```python
from build123d import *

# Parameters (mm, degrees)
BOSS_EXTRUDE1_DEPTH = 35
SKETCH5_R           = 1.5
BOSS_EXTRUDE2_DEPTH = 8.091605471
SKETCH6_R           = 1.5
CUT_EXTRUDE1_DEPTH  = 4


with BuildPart() as part:
    # Sketch3 → Boss-Extrude1 (new body)
    with BuildSketch(Plane(origin=(0, 0, 0), x_dir=(1, 0, 0), z_dir=(0, 1, 0))):
        Polygon((-3.464101615, 0), (-1.732050808, -3), (1.732050808, -3), (3.464101615, 0), (1.732050808, 3), (-1.732050808, 3), align=None)
    extrude(amount=BOSS_EXTRUDE1_DEPTH)

    # Sketch5 → Boss-Extrude2 (add)
    with BuildSketch(Plane(origin=(0, 35, 0), x_dir=(1, 0, 0), z_dir=(0, 1, 0))):
        with Locations(Location((0, 0, 0), (0, 0, 270))):
            Circle(SKETCH5_R)
    extrude(amount=BOSS_EXTRUDE2_DEPTH)

    # Sketch6 → Cut-Extrude1 (cut)
    with BuildSketch(Plane.XZ):
        with Locations(Location((0, 0, 0), (0, 0, 90))):
            Circle(SKETCH6_R)
    extrude(amount=-CUT_EXTRUDE1_DEPTH, mode=Mode.SUBTRACT)


solid = part.part
```
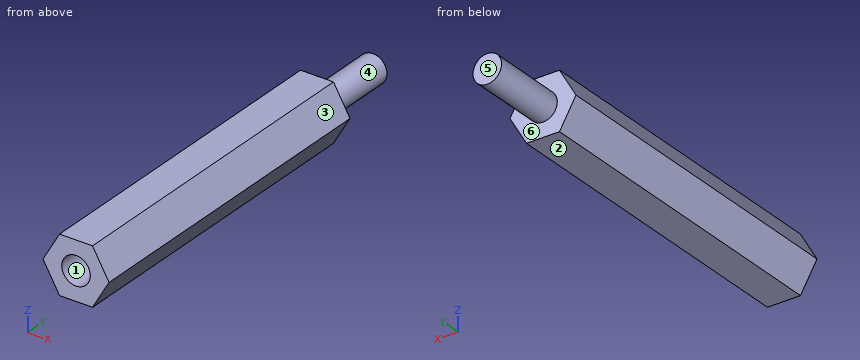
Can you work these out from the model? Positions are in its coordinate system, mm. Face numbers are marked on the shaded views. A direction names the side the tool comes from. Give positions to 0.01 mm unless a question says otherwise; leave off trailing zeros. Order: outer loops, then holes, each group sorted by start corner. A loop starts at its lowest first (then second) coordinate and runs counter-clockwise, first axis right, second up. Notation, with made-up numbers: M 56,-34.75 L 87,-34.75 A17 ccw 87,-1.75 Z; hole C -29.75,40 d4. An arc over 180 degrees is marked long. One line per item, written item: value.
1) I want a section at A-A, the plane x = 0. List the corners of the cut face in (y, z) for me.
Answer sheet:
outline: M 0,-3 L 35,-3 L 35,-1.5 L 43.09,-1.5 L 43.09,1.5 L 35,1.5 L 35,3 L 0,3 L 0,1.5 L 4,1.5 L 4,-1.5 L 0,-1.5 Z
2) I want a section at C-C, the plane z = 2. List the corners of the cut face in (x, y) for me, plus the area to 3 significant figures.
Answer sheet:
outline: M -2.31,0 L 2.31,0 L 2.31,35 L -2.31,35 Z
area: 162 mm^2
3) Please list where these lines run through material, in increasing order: line 1 along X through (y, z) = (1.45, 0); line 2 along Y through (x, z) = (2.75, 1); line 3 along Y through (x, z) = (-0.25, 0.75).
Answer sheet:
line 1: x = -3.46 to -1.5, 1.5 to 3.46
line 2: y = 0 to 35
line 3: y = 4 to 43.09
4) On a 3-axis mill with a long thin cutter (end or side, diameter ignored), from which of +Z, -Z, +X, -X, +Y, -Y can I reach the whole of each face in a straight line? I mean the marked faces 5 and 6. Say none if no direction works.
Answer sheet:
face 5: +Z, -Z, +X, -X, +Y
face 6: +Y
5) I want a section at D-D, the plane x = -3. List the corners of the cut face in (y, z) for me, plus the area to 3 significant figures.
Answer sheet:
outline: M 0,-0.8 L 35,-0.8 L 35,0.8 L 0,0.8 Z
area: 56.3 mm^2
6) For P1, Ø2, axis at x = -2.5, z = 1, coming from the +Y side, with a flat end and sliding along its axis, tell me the tip position at first contact or that it passes through.
Answer sheet:
P1: stops at y = 35
7) We'd pull the mould along X, two halves only. Please class the marked faces 1, 2, 3 and 4: released by +X, released by -X, zero draft, split by the parting line, or undercut.
Answer sheet:
face 1: undercut
face 2: zero draft
face 3: released by +X
face 4: split by the parting line
8) I want a section at B-B, the plane y = 34.5. List the corners of the cut face in (x, z) for me, plus the area to 3 significant figures.
Answer sheet:
outline: M -3.46,0 L -1.73,-3 L 1.73,-3 L 3.46,0 L 1.73,3 L -1.73,3 Z
area: 31.2 mm^2
